Build history of the part. All positions in model axes, mm. A direction names the side the tool comes from. Round coordinates to 2 decimals unless told otherwise and drop trailing zeros. Loops run counter-clockwise (first coordinate to the right, second up) from the corner with the lowest first, then second, coordinate; pieces in that order, holes last. Notation, with made-up numbers: M 58,-13 L 95,-13 A12 cw 95,-9 Z; hole C -23,-1.75 d8. An arc over 180 degrees is marked long. One line per item, written item: value.
```python
from build123d import *

# Parameters (mm, degrees)
BOSS_EXTRUDE1_DEPTH = 7
CUT_EXTRUDE1_REACH  = 49.215
SKETCH2_W           = 5.1
SKETCH2_H           = 3.1
CUT_EXTRUDE2_REACH  = 49.215
SKETCH3_R           = 2.1
FILLET1_START       = -1
FILLET1_DEPTH       = 9
FILLET1_2_DEPTH     = 7


with BuildPart() as part:
    # Sketch1 → Boss-Extrude1 (new body)
    with BuildSketch(Plane(origin=(0, 0, 0), x_dir=(1, 0, 0), z_dir=(0, 1, 0))):
        Polygon((0, 0), (18.2, 0), (18.2, 8), (5, 8), (5, 35), (8, 35), (8, 43), (0, 43), align=None)
    extrude(amount=BOSS_EXTRUDE1_DEPTH)

    # Sketch2 → Cut-Extrude1 (cut, up to next)
    with BuildSketch(Plane.XY, mode=Mode.PRIVATE) as cut_extrude1_sk1:
        with Locations((12.05, 3.5)):
            Rectangle(SKETCH2_W, SKETCH2_H)
    cut_extrude1_tool1 = extrude(cut_extrude1_sk1.sketch, amount=-CUT_EXTRUDE1_REACH, mode=Mode.PRIVATE) & part.part
    add(cut_extrude1_tool1.solids().sort_by_distance((12.05, 3.5, 0))[0], mode=Mode.SUBTRACT)

    # Sketch3 → Cut-Extrude2 (cut, up to next)
    with BuildSketch(Plane(origin=(0, 7, 0), x_dir=(1, 0, 0), z_dir=(0, 1, 0)), mode=Mode.PRIVATE) as cut_extrude2_sk1:
        with Locations(Location((4, 39, 0), (0, 0, 270))):
            Circle(SKETCH3_R)
    cut_extrude2_tool1 = extrude(cut_extrude2_sk1.sketch, amount=-CUT_EXTRUDE2_REACH, mode=Mode.PRIVATE) & part.part
    # Sketch3 → Cut-Extrude2 (cut, up to next)
    with BuildSketch(Plane(origin=(0, 7, 0), x_dir=(1, 0, 0), z_dir=(0, 1, 0)), mode=Mode.PRIVATE) as cut_extrude2_sk2:
        with Locations(Location((4, 4, 0), (0, 0, 270))):
            Circle(SKETCH3_R)
    cut_extrude2_tool2 = extrude(cut_extrude2_sk2.sketch, amount=-CUT_EXTRUDE2_REACH, mode=Mode.PRIVATE) & part.part
    add(cut_extrude2_tool1.solids().sort_by_distance((4, 7, -39))[0], mode=Mode.SUBTRACT)
    add(cut_extrude2_tool2.solids().sort_by_distance((4, 7, -4))[0], mode=Mode.SUBTRACT)

    # Fillet1: read off the stored shape, not the designer's step
    # Fillet1 outline → Fillet1 (cut)
    with BuildSketch(Plane(origin=(0, 0, 0), x_dir=(1, 0, 0), z_dir=(0, 1, 0)).offset(FILLET1_START)):
        with BuildLine():
            Line((18.2, 8), (16.7, 8))
            ThreePointArc((16.7, 8), (17.760660172, 7.560660172), (18.2, 6.5))
            Line((18.2, 6.5), (18.2, 8))
        make_face()
        with BuildLine():
            ThreePointArc((8, 36.5), (7.560660172, 35.439339828), (6.5, 35))
            Line((6.5, 35), (8, 35))
            Line((8, 35), (8, 36.5))
        make_face()
    extrude(amount=FILLET1_DEPTH, mode=Mode.SUBTRACT)

    # Fillet1 2 outline → Fillet1 2 (add)
    with BuildSketch(Plane(origin=(0, 0, 0), x_dir=(1, 0, 0), z_dir=(0, 1, 0))):
        with BuildLine():
            Line((5, 35), (5, 33.5))
            ThreePointArc((5, 33.5), (5.439339828, 34.560660172), (6.5, 35))
            Line((6.5, 35), (5, 35))
        make_face()
        with BuildLine():
            Line((5, 8), (6.5, 8))
            ThreePointArc((6.5, 8), (5.439339828, 8.439339828), (5, 9.5))
            Line((5, 9.5), (5, 8))
        make_face()
    extrude(amount=FILLET1_2_DEPTH)


solid = part.part
```
Item 1: Slice it at C-C, the plane z = -39. Give the cut face in (x, y).
Check values:
outline: M 0,0 L 1.9,0 L 1.9,7 L 0,7 Z; M 6.1,0 L 8,0 L 8,7 L 6.1,7 Z
Item 2: Slice it at D-D, the plane x = 10.75. Give the cut face in (y, z), and give its area (3 significant figures).
Check values:
outline: M 0,-8 L 1.95,-8 L 1.95,0 L 0,0 Z; M 5.05,-8 L 7,-8 L 7,0 L 5.05,0 Z
area: 31.2 mm2
Item 3: Wall check: line 1 along X through (y, z) = (4.5, -4); line 2 along X through (y, z) = (3.75, -3); line 3 along X through (y, z) = (5.5, -39). Give the ranges that are in metal, low to high.
Check values:
line 1: x = 0 to 1.9, 6.1 to 9.5, 14.6 to 18.2
line 2: x = 0 to 2.15, 5.85 to 9.5, 14.6 to 18.2
line 3: x = 0 to 1.9, 6.1 to 8
Item 4: Which spindle directions (+Z, -Z, +X, -X, +Y, -Y) get a long thin tool onto all of the face, cutting with end or side? Do faces 1 (the face through (12, 1.95, -4)), 2 (the face through (8, 3, -40)), 3 (the face through (18.2, 3, -3)), 4 (the face through (9, 3, -8)), 5 (the face through (4, 3, -43)). Say none if no direction does.
Check values:
face 1: +Z, -Z
face 2: -Z, +X, +Y, -Y
face 3: +Z, -Z, +X, +Y, -Y
face 4: +X, +Y, -Y
face 5: -Z, +X, -X, +Y, -Y
Item 5: Pull direction Y, two halves, no side cores. Call faces 6 (the face through (2.722, 3.549, -5.666)), 7 (the face through (14.6, 3, -4)), 8 (the face through (3, 7, -17)), 9 (the face through (12, 5.05, -4)): pulls with the +Y half, pulls with the -Y half, needs draft (parallel to the pull), parting line crosses it, or undercut.
Check values:
face 6: needs draft
face 7: undercut
face 8: pulls with the +Y half
face 9: undercut
Item 6: Slice it at B-B, the plane x = 4. Give the cut face in (y, z).
Check values:
outline: M 0,-43 L 7,-43 L 7,-41.1 L 0,-41.1 Z; M 0,-36.9 L 7,-36.9 L 7,-6.1 L 0,-6.1 Z; M 0,-1.9 L 7,-1.9 L 7,0 L 0,0 Z
Item 7: Slice it at A-A, the plane z = -4. Give the cut face in (x, y), and give its area (3 significant figures).
Check values:
outline: M 0,0 L 1.9,0 L 1.9,7 L 0,7 Z; M 6.1,0 L 18.2,0 L 18.2,7 L 6.1,7 Z; hole M 9.5,1.95 L 14.6,1.95 L 14.6,5.05 L 9.5,5.05 Z
area: 82.2 mm2
Item 8: Drop flat-ended pins along their axis: P1, Ø1.5, axis at y = 5, z = -12, coming from the +X side; P2, Ø2, axis at y = 3, z = -39.5, coming from the +X side. Give the stop position or say it passes through.
Check values:
P1: stops at x = 5
P2: stops at x = 8
